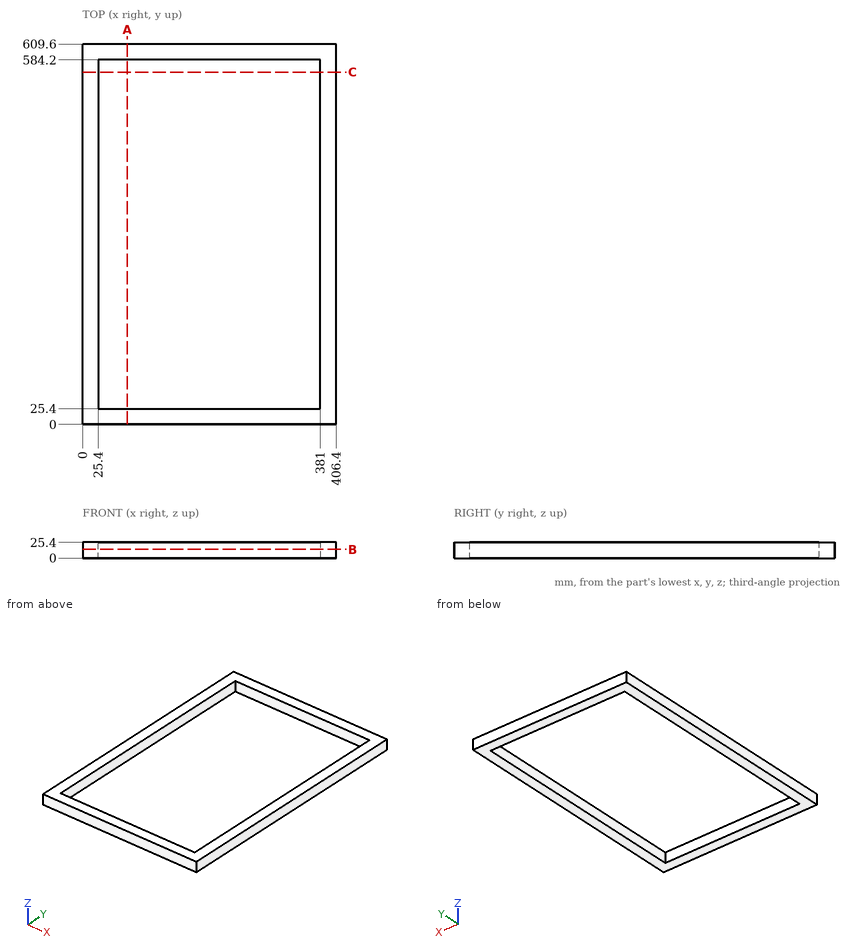
Source: three-view drawing plus pictorial views. Frame: mm from the lowest corner of the part. Round coordinates to 2 decimals unless told otherwise and drop trailing zeros. Loops run counter-clockwise (first coordinate to the right, second up) from the corner with the lowest first, then second, coordinate; pieces in that order, holes last.
Item 1: Section C-C, the plane y = 564.5. Output: boundary loops of the cut face in (x, z), plus the area to 3 significant figures.
Checked values:
outline: (0, 0) - (25.4, 0) - (25.4, 25.4) - (0, 25.4) - close; (381, 0) - (406.4, 0) - (406.4, 25.4) - (381, 25.4) - close
area: 1,290 mm2
Item 2: Section A-A, the plane x = 72. Output: boundary loops of the cut face in (y, z).
Checked values:
outline: (0, 0) - (25.4, 0) - (25.4, 25.4) - (0, 25.4) - close; (584.2, 0) - (609.6, 0) - (609.6, 25.4) - (584.2, 25.4) - close
Item 3: Section B-B, the plane z = 14.25. Output: boundary loops of the cut face in (x, y).
Checked values:
outline: (0, 0) - (406.4, 0) - (406.4, 609.6) - (0, 609.6) - close; hole (25.4, 25.4) - (381, 25.4) - (381, 584.2) - (25.4, 584.2) - close
Item 4: Line query: L1, parallel to X at y = 146.5, z = 14; L2, parallel to Y at x = 60.5, z = 10.5. Output: solid intervals per line, ascending.
Checked values:
L1: x = 0 to 25.4, 381 to 406.4
L2: y = 0 to 25.4, 584.2 to 609.6
